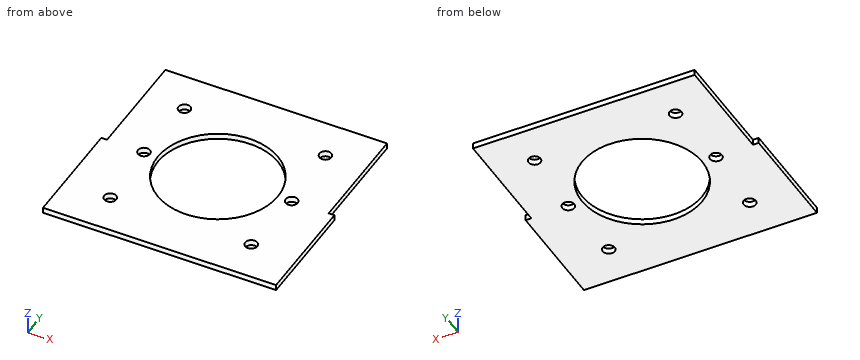
```python
from build123d import *

# Parameters (mm, degrees)
SKETCH1_W           = 120
SKETCH1_H           = 120
SKETCH1_R           = 3.25
BOSS_EXTRUDE1_DEPTH = 3.1
SKETCH2_W           = 3.1
SKETCH2_H           = 60
BOSS_EXTRUDE3_DEPTH = 3.1
SKETCH5_R           = 32.5
CUT_EXTRUDE2_DEPTH  = 4.1


with BuildPart() as part:
    # Sketch1 → Boss-Extrude1 (new body)
    with BuildSketch(Plane.XY):
        Rectangle(SKETCH1_W, SKETCH1_H)
        with Locations((-38.166088515, 38.166088515)):
            Circle(SKETCH1_R, mode=Mode.SUBTRACT)
        with Locations((38.166088515, 38.166088515)):
            Circle(SKETCH1_R, mode=Mode.SUBTRACT)
        with Locations((38.166088515, -38.166088515)):
            Circle(SKETCH1_R, mode=Mode.SUBTRACT)
        with Locations((-38.166088515, -38.166088515)):
            Circle(SKETCH1_R, mode=Mode.SUBTRACT)
        with Locations((-40, 0)):
            Circle(SKETCH1_R, mode=Mode.SUBTRACT)
        with Locations((40, 0)):
            Circle(SKETCH1_R, mode=Mode.SUBTRACT)
    extrude(amount=BOSS_EXTRUDE1_DEPTH)

    # Sketch2 → Boss-Extrude3 (add, through all)
    with BuildSketch(Plane.XY.offset(3.1)):
        with Locations((61.55, -30)):
            Rectangle(SKETCH2_W, SKETCH2_H)
        with Locations((-61.55, -30)):
            Rectangle(SKETCH2_W, SKETCH2_H)
    extrude(amount=-BOSS_EXTRUDE3_DEPTH)

    # Sketch5 → Cut-Extrude2 (cut, through all)
    with BuildSketch(Plane.XY.offset(3.1)):
        Circle(SKETCH5_R)
    extrude(amount=-CUT_EXTRUDE2_DEPTH, mode=Mode.SUBTRACT)


solid = part.part
```
Build history of the part. All positions in model axes, mm. Coordinates: 2 decimals unless noted, no trailing zeros. Write each loop counter-clockwise with the first axis right and the second up, starting at its lowest first coordinate (ties: lowest second). Pieces come first, ordered by that corner, then holes.
1. Band-saw the part on D-D, the plane z = 0.6. Give the cut face in (x, y).
Answer block:
outline: (-63.1, -60) - (63.1, -60) - (63.1, 0) - (60, 0) - (60, 60) - (-60, 60) - (-60, 0) - (-63.1, 0) - close; hole circle Ø6.5 at (-40, 0); hole circle Ø6.5 at (-38.17, -38.17); hole circle Ø6.5 at (-38.17, 38.17); hole circle Ø65 at (0, 0); hole circle Ø6.5 at (38.17, -38.17); hole circle Ø6.5 at (38.17, 38.17); hole circle Ø6.5 at (40, 0)
2. Band-saw the part on C-C, the plane x = 40. Give the cut face in (y, z).
Answer block:
outline: (-60, 0) - (-40.85, 0) - (-40.85, 3.1) - (-60, 3.1) - close; (-35.48, 0) - (-3.25, 0) - (-3.25, 3.1) - (-35.48, 3.1) - close; (3.25, 0) - (35.48, 0) - (35.48, 3.1) - (3.25, 3.1) - close; (40.85, 0) - (60, 0) - (60, 3.1) - (40.85, 3.1) - close
3. Drop flat-ended pins along their axis: pin 1 (0.9 mm diameter, centred on y = 38, z = 1, fed in from +X); pin 2 (0.9 mm diameter, centred on y = 26.5, z = 1.5, fed in from -X). Give the stop position or say it passes through.
Answer block:
pin 1: stops at x = 60
pin 2: stops at x = -60
4. Band-saw the part on A-A, the plane x = 0. Give the cut face in (y, z), and give its area (4 significant figures).
Answer block:
outline: (-60, 0) - (-32.5, 0) - (-32.5, 3.1) - (-60, 3.1) - close; (32.5, 0) - (60, 0) - (60, 3.1) - (32.5, 3.1) - close
area: 170.5 mm2
5. Band-saw the part on B-B, the plane y = -7.5. Give the cut face in (x, z), and give its area (3 significant figures).
Answer block:
outline: (-63.1, 0) - (-31.62, 0) - (-31.62, 3.1) - (-63.1, 3.1) - close; (31.62, 0) - (63.1, 0) - (63.1, 3.1) - (31.62, 3.1) - close
area: 195 mm2
6. Drill centre lines: probe 1 along Y at (x, z) = (0, 1.45); probe 2 along X at (y, z) = (35.5, 0.95); probe 3 along X at (y, z) = (38.5, 2.5). Where is each one in solid material? Low to high.
Answer block:
probe 1: y = -60 to -32.5, 32.5 to 60
probe 2: x = -60 to -40.02, -36.31 to 36.31, 40.02 to 60
probe 3: x = -60 to -41.4, -34.93 to 34.93, 41.4 to 60
